Work out the finished part from the listing and answer in its coordinate system (mm). A direction names the side the tool comes from. Round coordinates to 2 decimals unless told otherwise and drop trailing zeros. Write each loop counter-clockwise with the first axis right and the second up, starting at its lowest first coordinate (ties: lowest second). Pieces come first, ordered by that corner, then holes.
Autodesk Inventor part; units mm, degrees
ref_plane "YZ Plane" through (0, 0, 0) normal (1, 0, 0) x (0, 1, 0)
ref_plane "XZ Plane" through (0, 0, 0) normal (0, 1, 0) x (-1, 0, 0)
ref_plane "XY Plane" through (0, 0, 0) normal (0, 0, 1) x (1, 0, 0)
sketch "Sketch1" plane through (0, 0, 0) normal (0, 1, 0) x (-1, 0, 0)
  line L0 (0, 0) -> (100, 0)
  line L1 (100, 0) -> (100, -100)
  line L2 (100, -100) -> (0, -100)
  line L3 (0, -100) -> (0, 0)
  dimension "d0" = 100
  dimension "d1" = 100
extrude "Extrusion1" add sketch "Sketch1" along normal blind 30
sketch "Sketch2" plane through (0, 30, 0) normal (0, 1, 0) x (1, 0, 0)
  line L0 (0, 0) -> (0, 100)
  line L1 (-100, 0) -> (0, 0)
  line L2 (0, 10) -> (0, 0)
  line L3 (-10, 10) -> (-90, 10)
  line L4 (-90, 10) -> (-90, 90)
  line L5 (-90, 90) -> (-10, 90)
  line L6 (-10, 90) -> (-10, 10)
  dimension "d6" = 80
  dimension "d7" = 80
extrude "Extrusion2" cut sketch "Sketch2" against normal blind 20
sketch "Sketch5" plane through (0, 0, 0) normal (1, 0, 0) x (0, 0, -1)
  point P0 (0, 0)
sketch "Sketch6" plane through (0, 0, 0) normal (1, 0, 0) x (0, 0, -1)
  line L0 (13, 16) -> (15, 16)
  line L1 (15, 16) -> (15, 14)
  line L2 (15, 14) -> (13, 14)
  line L3 (13, 14) -> (13, 16)
  line L4 (13, 16) -> (15, 14) construction
  line L5 (15, 16) -> (13, 14) construction
  line L6 (85, 16) -> (87, 16)
  line L7 (87, 16) -> (87, 14)
  line L8 (87, 14) -> (85, 14)
  line L9 (85, 14) -> (85, 16)
  line L10 (85, 16) -> (87, 14) construction
  line L11 (87, 16) -> (85, 14) construction
  point P0 (0, 0)
  point P1 (14, 15)
  point P2 (86, 15)
  dimension "d22" = 2
  dimension "d23" = 2
  dimension "d24" = 2
  dimension "d25" = 2
extrude "Extrusion5" add sketch "Sketch6" along normal blind 15
pattern_linear "Rectangular Pattern1" count 2 spacing 115 along (-1, 0, 0) of "Extrusion5"
sketch "Sketch7" plane through (0, 16, -85) normal (0, 1, 0) x (1, 0, 0)
  circle A0 centre (13, 1) radius 0.75
  point P0 (0, -85)
  dimension "d31" = 1.5
extrude "Extrusion6" add sketch "Sketch7" along normal blind 55
sketch "Sketch8" plane through (0, 14, -87) normal (0, -1, 0) x (1, 0, 0)
  circle A0 centre (13, 1) radius 0.75
  circle A1 centre (13, 1) radius 0.75
  point P0 (0, 87)
  dimension "d34" = 1.5
extrude "Extrusion7" add sketch "Sketch8" along normal blind 2
thread "Thread1"
pattern_linear "Rectangular Pattern2" count 2 spacing 72 along (0, 0, 1) of "Extrusion6"
pattern_linear "Rectangular Pattern3" count 2 spacing 126 along (-1, 0, 0) of "Extrusion6", "Rectangular Pattern2"
thread "Thread2"
thread "Thread3"
thread "Thread4"
pattern_linear "Rectangular Pattern4" count 2 spacing 72 along (0, 0, 1) count 2 spacing 126 along (-1, 0, 0) of "Extrusion7"
thread "Thread5"
thread "Thread6"
thread "Thread7"
sketch "Sketch9" plane through (-100, 0, -100) normal (-1, 0, 0) x (0, 0, 1)
  point P0 (100, 0)
sketch "Sketch10" plane through (-113, 71, -14) normal (0, 1, 0) x (1, 0, 0)
  point P0 (113, -14)
sketch "Sketch11" plane through (-113, 71, -86) normal (0, 1, 0) x (1, 0, 0)
  line L0 (-2, -1) -> (-2, 1)
  line L1 (-2, 1) -> (16, 1)
  line L2 (16, 1) -> (16, -1)
  line L3 (16, -1) -> (-2, -1)
  line L4 (-2, -1) -> (-2, 1)
  point P0 (113, -86)
  dimension "d63" = 18
extrude "Extrusion8" add sketch "Sketch11" along normal blind 2
sketch "Sketch12" plane through (-113, 73, -86) normal (0, 1, 0) x (1, 0, 0)
  point P0 (113, -86)
sketch "Sketch13" plane through (13, 71, -86) normal (0, 1, 0) x (1, 0, 0)
  line L0 (-13, -1) -> (2, -1)
  line L1 (2, -1) -> (-16, -1)
  line L2 (-16, -1) -> (-16, 1)
  line L3 (-16, 1) -> (2, 1)
  line L4 (2, 1) -> (2, -1)
  point P0 (-13, -86)
  dimension "d66" = 18
  dimension "d67" = 2
extrude "Extrusion9" add sketch "Sketch13" along normal blind 2
pattern_linear "Rectangular Pattern5" count 2 spacing 72 along (0, 0, 1) of "Extrusion9"
pattern_linear "Rectangular Pattern6" count 2 spacing 72 along (0, 0, 1) of "Extrusion8"
properties part number "container 1" material "Silver"
Q1. Find the intervals of material crossed by L1, parallel to X at y = 13.5, z = -43.5; L2, parallel to Y at x = -41.5, z = -40.5, in increasing order.
Q2. Find section B-B (x = -80.5). Determine the outline of the cut face in (y, z).
Q3. The mould has two halves that part along Z. Classify faces 1 (the face through (-51, 15, -100)), 2 (the face through (-90, 20, -49)), 3 (the face through (-49, 15, 0)): +Z half, -Z half, draft (parallel to the pull), parting line (faces both ways), or undercut.
Q4. Find section A-A (y = 23). Determine the outline of the cut face in (x, z).
Q5. Find section D-D (z = -37). Determine the outline of the cut face in (x, y).
Q6. A tool of negligible diameter and unlimited length cuts with its end or side. For faces 4 (the face through (-51, 20, -90)), 5 (the face through (-49, 0, -49)), from which of +Z, -Z, +X, -X, +Y, -Y can it reach the whole face along a straight path? Write none if from no direction.
Q7. Given pin 1 (1 mm diameter, centred on x = -107, y = 72, fed in from +Z); pin 2 (12 mm diameter, centred on x = -76, y = 22.5, fed in from +Z); pin 3 (22 mm diameter, centred on y = 23.5, z = -56.5, fed in from -X); pin 4 (1.2 mm diameter, centred on x = -113, z = -14.5, fed in from -Y), each flat-ended and moving along its own axis, determine where each tip first touches the part or whether it passes through.
Q8. Find section C-C (y = 38). Determine the outline of the cut face in (x, z).
Report:
1. L1: x = -100 to -90, -10 to 0
1. L2: y = 0 to 10
2. outline: (0, -100) - (30, -100) - (30, -90) - (10, -90) - (10, -10) - (30, -10) - (30, 0) - (0, 0) - close
3. face 1: -Z half
3. face 2: undercut
3. face 3: +Z half
4. outline: circle Ø1.5 at (-113, -86); circle Ø1.5 at (-113, -14); (-100, -100) - (0, -100) - (0, 0) - (-100, 0) - close; circle Ø1.5 at (13, -86); circle Ø1.5 at (13, -14); hole (-90, -90) - (-10, -90) - (-10, -10) - (-90, -10) - close
5. outline: (-100, 0) - (0, 0) - (0, 30) - (-10, 30) - (-10, 10) - (-90, 10) - (-90, 30) - (-100, 30) - close
6. face 4: +Y
6. face 5: +Z, -Z, +X, -X, -Y
7. pin 1: stops at z = -13
7. pin 2: stops at z = 0
7. pin 3: stops at x = -100
7. pin 4: stops at y = 12
8. outline: circle Ø1.5 at (-113, -86); circle Ø1.5 at (-113, -14); circle Ø1.5 at (13, -86); circle Ø1.5 at (13, -14)
